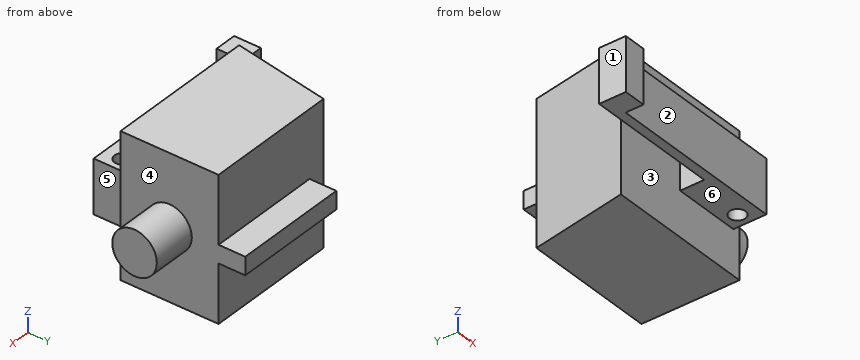
from build123d import *

# Parameters (mm, degrees)
F1_DEPTH  = 18
F2_R      = 2.5
F3_DEPTH  = 5
F4_W      = 13
F4_H      = 2
F5_DEPTH  = 3
F6_W      = 7.5974241367
F6_H      = 6
F7_DEPTH  = 3.7
F8_R      = 0.9
F9_DEPTH  = 10
F10_W     = 1
F10_H     = 6
F11_DEPTH = 15
F12_W     = 2.5
F12_H     = 6
F13_DEPTH = 2
F14_DEPTH = 1
F15_DEPTH = 1


with BuildPart() as f1:
    # F0 (on Top) → F1 (new body)
    with BuildSketch(Plane.XY):
        Polygon((-2.5732557046, 7.6509772142), (-17.5732557046, 7.6509772142), (-19.5128524924, -3.3490227858), (-2.5732557046, -3.3490227858), align=None)
    extrude(amount=F1_DEPTH)

    # F2 (on face) → F3 (join)
    with BuildSketch(Plane.YZ.offset(-2.5732557046)):
        with Locations((2.1509772142, 9)):
            Circle(F2_R)
    extrude(amount=F3_DEPTH)

    # F4 (on face) → F5 (join)
    with BuildSketch(Plane(origin=(0, 7.6509772142, 0), x_dir=(-1, 0, 0), z_dir=(0, 1, 0))):
        with Locations((9.0732557046, 8.5)):
            Rectangle(F4_W, F4_H)
    extrude(amount=F5_DEPTH)

    # F6 (on face) → F7 (join)
    with BuildSketch(Plane.XZ.offset(3.3490227858)):
        with Locations((-7.2443420301, 9)):
            Rectangle(F6_W, F6_H)
    extrude(amount=F7_DEPTH)

    # F8 (on face) → F9 (cut)
    with BuildSketch(Plane.XY.offset(12)):
        with Locations((-4.9705179408, -5.0118290819)):
            Circle(F8_R)
    extrude(amount=-F9_DEPTH, mode=Mode.SUBTRACT)

    # F10 (on face) → F11 (join)
    with BuildSketch(Plane(origin=(-11.0430540985, 0, 0), x_dir=(0, -1, 0), z_dir=(-1, 0, 0))):
        with Locations((6.5490227858, 9)):
            Rectangle(F10_W, F10_H)
    extrude(amount=F11_DEPTH)

    # F12 (on face) → F13 (join)
    with BuildSketch(Plane.XZ.offset(7.0490227858)):
        with Locations((-24.7930540985, 9)):
            Rectangle(F12_W, F12_H)
    extrude(amount=F13_DEPTH)

    # F14 (cut): a face of the model
    f14_faces = [f1.faces().sort_by_distance(p)[0] for p in [
        (-10.5679703972, 2.0396443295, 0),
    ]]
    extrude(f14_faces, amount=-F14_DEPTH, mode=Mode.SUBTRACT)

    # F15 (cut): a face of the model
    f15_faces = [f1.faces().sort_by_distance(p)[0] for p in [
        (-10.5679703972, 2.0396443295, 18),
    ]]
    extrude(f15_faces, amount=-F15_DEPTH, mode=Mode.SUBTRACT)


solid = f1.part
Geometry: final body of the model. Coordinates: model frame, mm. Face numbers are marked on the shaded views. A direction names the side the tool comes from. Coordinates: 2 decimals unless noted, no trailing zeros. Order: outer loops, then holes, each group sorted by start corner. A loop starts at its lowest first (then second) coordinate and runs counter-clockwise, first axis right, second up.
1) Set-up query: the marked faces 4, 5 and 6. Return all of +Z, -Z, +X, -X, +Y, -Y with unobstructed straight access to the full face (end or side cutting, diameter ignored); none if empty.
Result sheet:
face 4: +X
face 5: +Z, -Z, +X, -Y
face 6: -Z, +X, -X, -Y
2) Section C-C (x = -8). Return loops of the section in (y, z), then the cut area to 3 significant figures.
Result sheet:
outline: (-7.05, 6) - (-3.35, 6) - (-3.35, 1) - (7.65, 1) - (7.65, 7.5) - (10.65, 7.5) - (10.65, 9.5) - (7.65, 9.5) - (7.65, 17) - (-3.35, 17) - (-3.35, 12) - (-7.05, 12) - close
area: 204 mm2
3) Section A-A (x = -13.5). Return loops of the section in (y, z).
Result sheet:
outline: (-7.05, 6) - (-6.05, 6) - (-6.05, 12) - (-7.05, 12) - close; (-3.35, 1) - (7.65, 1) - (7.65, 7.5) - (10.65, 7.5) - (10.65, 9.5) - (7.65, 9.5) - (7.65, 17) - (-3.35, 17) - close
4) Draft query along Y for the marked faces 1, 2 and 3. Return one class per face: released by +Y, released by -Y, zero draft, split by the parting line, or undercut.
Result sheet:
face 1: zero draft
face 2: released by -Y
face 3: undercut
5) Ray query, probe 1 along Y at (x, z) = (-14.75, 6.25); probe 2 along Y at (x, z) = (-3.75, 9.25); probe 3 along Z at (x, y) = (-10.75, 9.25). Return the intervals inside material, ascending.
Result sheet:
probe 1: y = -7.05 to -6.05, -3.35 to 7.65
probe 2: y = -7.05 to 10.65
probe 3: z = 7.5 to 9.5
6) First-contact query: P1, Ø2, axis at y = 10, z = 8, coming from the -X side; P2, Ø6.5, axis at x = -16.5, y = -7, coming from the -Z side; P3, Ø3, axis at x = -9.5, y = -7, coming from the +Z side; P4, Ø8, axis at y = -6, z = 12, coming from the -X side. Flat tips, straight axial feed; report the tip coordinate or a pass-through.
Result sheet:
P1: stops at x = -15.57
P2: stops at z = 6
P3: stops at z = 12
P4: stops at x = -26.04
7) Section B-B (z = 7). Return loops of the section in (x, y).
Result sheet:
outline: (-26.04, -9.05) - (-23.54, -9.05) - (-23.54, -7.05) - (-3.45, -7.05) - (-3.45, -3.35) - (-2.57, -3.35) - (-2.57, 0.65) - (2.43, 0.65) - (2.43, 3.65) - (-2.57, 3.65) - (-2.57, 7.65) - (-17.57, 7.65) - (-19.51, -3.35) - (-11.04, -3.35) - (-11.04, -6.05) - (-26.04, -6.05) - close; hole circle Ø1.8 at (-4.97, -5.01)
8) Section D-D (y = 1). Return loops of the section in (x, z), then the cut area to 3 significant figures.
Result sheet:
outline: (-18.75, 1) - (-2.57, 1) - (-2.57, 6.78) - (2.43, 6.78) - (2.43, 11.22) - (-2.57, 11.22) - (-2.57, 17) - (-18.75, 17) - close
area: 281 mm2
